```python
from build123d import *

# Parameters (mm, degrees)
SKETCH_1_R      = 1.5
EXTRUDE_1_DEPTH = 2
FILLET_1_R      = 1


with BuildPart() as part:
    # 草图1 → 凸台-拉伸1 (new body)
    with BuildSketch(Plane.XY):
        Polygon((-133.240644315, -50.984206154), (-133.240644315, -37.984206154), (-125.740644315, -24.993825098), (-117.080390278, -29.993825098), (-113.240644315, -40.984206154), (-113.240644315, -50.984206154), (-123.240644315, -50.984206154), align=None)
        with Locations((-128.240644315, -45.984206154)):
            Circle(SKETCH_1_R, mode=Mode.SUBTRACT)
        with Locations((-123.910517296, -31.823952117)):
            Circle(SKETCH_1_R, mode=Mode.SUBTRACT)
        with Locations((-118.240644315, -45.984206154)):
            Circle(SKETCH_1_R, mode=Mode.SUBTRACT)
    extrude(amount=EXTRUDE_1_DEPTH)

    # 圆角1
    fillet_1_edges = [part.edges().sort_by_distance(p)[0] for p in [
        (-133.240644315, -50.984206154, 1),
        (-133.240644315, -37.984206154, 1),
        (-125.740644315, -24.993825098, 1),
        (-117.080390278, -29.993825098, 1),
        (-113.240644315, -40.984206154, 1),
        (-113.240644315, -50.984206154, 1),
    ]]
    fillet(fillet_1_edges, radius=FILLET_1_R)


solid = part.part
```
Verification items for the finished model (mm, model axes). Round coordinates to 2 decimals unless told otherwise and drop trailing zeros. Write each loop counter-clockwise with the first axis right and the second up, starting at its lowest first coordinate (ties: lowest second). Pieces come first, ordered by that corner, then holes. Notation, with made-up numbers: (57.5, 71.25) -> (78.5, 71.25) arc R16 cw to (78.5, 77.25) -> close; hole circle Ø3 at (60, -18.5). An arc over 180 degrees is marked (long way). Write each question's results on one line, items separated by ' | '.
Q1. Go/stop test with a flat-tipped pin: pin 1 Ø6 at (x, y) = (-116, -30.5) entering from -Z. Record where the tip stops, or that it passes through.
Derived:
pin 1: stops at z = 0
Q2. Sectioned sample at B-B, the plane x = -118.75. Record the boundary of the cut face in (y, z).
Derived:
outline: (-50.98, 0) -> (-47.4, 0) -> (-47.4, 2) -> (-50.98, 2) -> close; (-44.57, 0) -> (-29.03, 0) -> (-29.03, 2) -> (-44.57, 2) -> close
Q3. Draft check along Y on faces 1 (the face through (-126.81, -45.53, 0.99)), 2 (the face through (-113.241, -46, 1)), 3 (the face through (-113.54, -50.7, 1.01)). Enter one of: released by +Y, released by -Y, zero draft, split by the parting line, or undercut.
Derived:
face 1: undercut | face 2: zero draft | face 3: released by -Y
Q4. Sectioned sample at A-A, the plane y = -44.75. Record the boundary of the cut face in (x, z), and give its area (3 significant figures).
Derived:
outline: (-133.24, 0) -> (-129.09, 0) -> (-129.09, 2) -> (-133.24, 2) -> close; (-127.39, 0) -> (-119.09, 0) -> (-119.09, 2) -> (-127.39, 2) -> close; (-117.39, 0) -> (-113.24, 0) -> (-113.24, 2) -> (-117.39, 2) -> close | area: 33.2 mm²
Q5. Sectioned sample at D-D, the plane x = -121.75. Record the boundary of the cut face in (y, z).
Derived:
outline: (-50.98, 0) -> (-27.3, 0) -> (-27.3, 2) -> (-50.98, 2) -> close
Q6. Sectioned sample at C-C, the plane z = 1.5. Record the boundary of the cut face in (x, y).
Derived:
outline: (-133.24, -49.98) arc R1 ccw to (-132.24, -50.98) -> (-114.24, -50.98) arc R1 ccw to (-113.24, -49.98) -> (-113.24, -41.15) arc R1 ccw to (-113.3, -40.82) -> (-116.96, -30.34) arc R1 ccw to (-117.4, -29.81) -> (-124.87, -25.49) arc R1 ccw to (-126.24, -25.86) -> (-133.11, -37.75) arc R1 ccw to (-133.24, -38.25) -> close; hole circle Ø3 at (-128.24, -45.98); hole circle Ø3 at (-123.91, -31.82); hole circle Ø3 at (-118.24, -45.98)
Q7. Thickness scan on probe 1 along X at (y, z) = (-45, 1); probe 2 along Y at (x, z) = (-127.25, 0.75); probe 3 along Y at (x, z) = (-123.5, 0.15). Record the ranges inside material, lowest first.
Derived:
probe 1: x = -133.24 to -129.37, -127.11 to -119.37, -117.11 to -113.24 | probe 2: y = -50.98 to -47.11, -44.86 to -27.61 | probe 3: y = -50.98 to -33.27, -30.38 to -26.29
